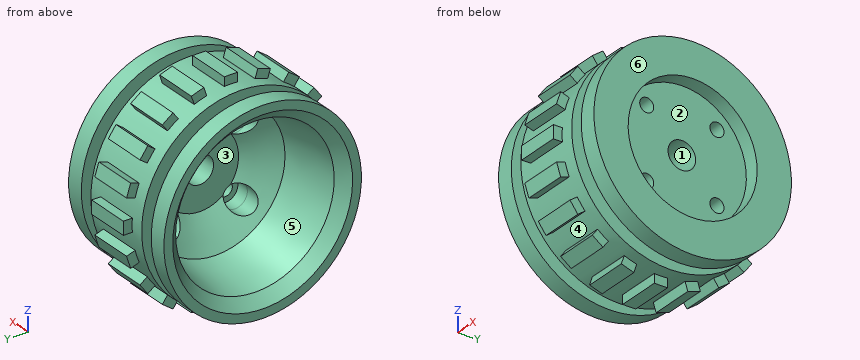
```python
from build123d import *

# Parameters (mm, degrees)
SKETCH_5_R               = 1.6
CUT_EXTRUDE_1_DEPTH      = 42.473606065
SKETCH_6_R               = 2.85
CUT_EXTRUDE_2_DEPTH      = 3
CHAMFER_1_SIZE           = 5
CHAMFER_1_SIZE_2         = 6.164015259
CHAMFER_2_SIZE           = 2
CHAMFER_2_SIZE2          = 2.465606104
SKETCH_8_W               = 3
SKETCH_8_H               = 4
SKETCH_56_W              = 10
SKETCH_56_H              = 3.522984106
EXTRUDE_2_DEPTH          = 1.5
PATTERN_CIRCULAR_2_COUNT = 20


with BuildPart() as part:
    # Эскиз4 → Повернуть1 (revolve)
    with BuildSketch(Plane.XY, mode=Mode.PRIVATE) as revolve_1_sk:
        Polygon((-30, 22.5), (-30, 18.491274218), (-10.2, 15), (-10.2, 3.15), (-3.4, 3.15), (-3.4, 14.7), (0, 14.7), (0, 22.5), align=None)
    revolve(revolve_1_sk.sketch.rotate(Axis((-30, 0, 0), (1, 0, 0)), 90), axis=Axis((-30, 0, 0), (1, 0, 0)))

    # Эскиз5 → Вырез-Вытянуть1 (cut, through all)
    with BuildSketch(Plane(origin=(-3.4, 0, 0), x_dir=(0, 0, -1), z_dir=(1, 0, 0))):
        with Locations((8.000913229, 8.000913229)):
            Circle(SKETCH_5_R)
        with Locations((-8.000913229, 8.000913229)):
            Circle(SKETCH_5_R)
        with Locations((-8.000913229, -8.000913229)):
            Circle(SKETCH_5_R)
        with Locations((8.000913229, -8.000913229)):
            Circle(SKETCH_5_R)
    extrude(amount=-CUT_EXTRUDE_1_DEPTH, mode=Mode.SUBTRACT)

    # Эскиз6 → Вырез-Вытянуть2 (cut)
    with BuildSketch(Plane.ZY.offset(10.2)):
        with Locations((-8.000913229, 8.000913229)):
            Circle(SKETCH_6_R)
        with Locations((8.000913229, 8.000913229)):
            Circle(SKETCH_6_R)
        with Locations((8.000913229, -8.000913229)):
            Circle(SKETCH_6_R)
        with Locations((-8.000913229, -8.000913229)):
            Circle(SKETCH_6_R)
    extrude(amount=-CUT_EXTRUDE_2_DEPTH, mode=Mode.SUBTRACT)

    # Фаска1
    # the kernel refuses this chamfer: 6.164015259, 5 mm, written as the material it adds along each edge
    with BuildSketch(Plane(origin=(-10.2, 0, 0), x_dir=(0, 0, 1), z_dir=(0, 1, 0))) as chamfer_1_piece_1_section:
        Polygon((15 + CHAMFER_1_SIZE * 0.173648177667, -CHAMFER_1_SIZE * 0.984807753012), (15 - CHAMFER_1_SIZE_2, 0), (15, 0), align=None)
    chamfer_1_piece_1 = revolve(axis=Axis((-10.2, 0, 0), (1, 0, 0)), mode=Mode.PRIVATE)
    chamfer_1_piece_1 = chamfer_1_piece_1 - Plane(origin=(-12.574838132, 8.000913229, -8.000913229), x_dir=(0, 0, 1), z_dir=(-1, 0, 0)) * Cylinder(2.85, 64, mode=Mode.PRIVATE)
    chamfer_1_piece_1 = chamfer_1_piece_1 - Plane(origin=(-12.574838132, 8.000913229, 8.000913229), x_dir=(0, 0, 1), z_dir=(-1, 0, 0)) * Cylinder(2.85, 64, mode=Mode.PRIVATE)
    chamfer_1_piece_1 = chamfer_1_piece_1 - Plane(origin=(-12.574838132, -8.000913229, -8.000913229), x_dir=(0, 0, 1), z_dir=(-1, 0, 0)) * Cylinder(2.85, 64, mode=Mode.PRIVATE)
    chamfer_1_piece_1 = chamfer_1_piece_1 - Plane(origin=(-12.574838132, -8.000913229, 8.000913229), x_dir=(0, 0, 1), z_dir=(-1, 0, 0)) * Cylinder(2.85, 64, mode=Mode.PRIVATE)
    add(chamfer_1_piece_1)

    # Фаска2
    chamfer_2_edges = [part.edges().sort_by_distance(p)[0] for p in [
        (-30, 0, -18.491274218),
    ]]
    chamfer_2_side = [part.faces().sort_by_distance(p)[0] for p in [
        (-30, 0, -21.863603897),
    ]]
    chamfer(chamfer_2_edges, length=CHAMFER_2_SIZE, length2=CHAMFER_2_SIZE2, reference=chamfer_2_side[0])

    # Эскиз8 → Вырез-Повернуть1 (revolve, cut)
    with BuildSketch(Plane.XY, mode=Mode.PRIVATE) as cut_revolve_1_sk:
        with Locations((-24.5, 21.5)):
            Rectangle(SKETCH_8_W, SKETCH_8_H)
        with Locations((-5.5, 21.5)):
            Rectangle(SKETCH_8_W, SKETCH_8_H)
    revolve(cut_revolve_1_sk.sketch.rotate(Axis((-30, 0, 0), (1, 0, 0)), 90), axis=Axis((-30, 0, 0), (1, 0, 0)), mode=Mode.SUBTRACT)

    # Эскиз56 → Бобышка-Вытянуть2 (add, symmetric)
    with BuildSketch(Plane.XY):
        with Locations((-15, 22.738507947)):
            Rectangle(SKETCH_56_W, SKETCH_56_H)
    extrude_2 = extrude(amount=EXTRUDE_2_DEPTH, both=True)

    # Круговой массив2: Бобышка-Вытянуть2 ×20 about axis
    pattern_circular_2_axis = Axis((0, 0, 0), (1, 0, 0))
    for i in range(1, PATTERN_CIRCULAR_2_COUNT):
        add(extrude_2.rotate(pattern_circular_2_axis, i * 360 / PATTERN_CIRCULAR_2_COUNT))


solid = part.part
```
For this review, take the finished solid that the model builds, in its own axes (mm). Face numbers are marked on the shaded views. A direction names the side the tool comes from. Round coordinates to 2 decimals unless told otherwise and drop trailing zeros. Write each loop counter-clockwise with the first axis right and the second up, starting at its lowest first coordinate (ties: lowest second). Pieces come first, ordered by that corner, then holes. Notation, with made-up numbers: (73.5, 10.25) -> (82.5, 10.25) arc R23 cw to (82.5, 19.25) -> close; hole circle Ø9 at (79, 10.5). An arc over 180 degrees is marked (long way). One line per question, with ' | ' between items. Start each with the question number.
1) Mouldability with a two-part tool opening along Z and no side actions: class the marked faces 5 and 6 as +Z half, -Z half, draft (parallel to the pull), parting line (faces both ways), or undercut.
2) Add section A-A (x = -6.25). Write out the cut boundary in (y, z).
3) Machinability: for the marked faces 1, 2, 3 and 4, which of the approach directions +Z, -Z, +X, -X, +Y, -Y give a long, thin tool a straight path to every point of the face, cutting with its end or side? Answer none if there is none.
4) For pin 1 Ø10 at (x, z) = (-21, -9) entering from -Y; pin 2 Ø6 at (x, z) = (-18, -16.5) entering from +Y; pin 3 Ø4 at (y, z) = (18.5, -13) entering from -X; pin 4 Ø6 at (y, z) = (6, 2) entering from -X, all flat-tipped, find the tip position at first contact; note any pin that passes through.
5) Wall thickness on line 1 along X through (y, z) = (6, 20); line 2 along Y through (x, z) = (-18.5, -19.5); line 3 along Y through (x, z) = (-7.25, -5.5): over which ranges is each line inside the solid? List them lowest first.
Reported:
1) face 5: undercut | face 6: draft
2) outline: circle Ø39 at (0, 0); hole circle Ø3.2 at (-8, -8); hole circle Ø3.2 at (-8, 8); hole circle Ø6.3 at (0, 0); hole circle Ø3.2 at (8, -8); hole circle Ø3.2 at (8, 8)
3) face 1: +X, -X | face 2: +X | face 3: -X | face 4: none
4) pin 1: stops at y = -23.76 | pin 2: stops at y = 20.48 | pin 3: stops at x = -30 | pin 4: stops at x = -10.54
5) line 1: x = -30 to -26, -23 to -7, -4 to 0 | line 2: y = -14.84 to -12.31, -11.22 to 11.22, 12.31 to 14.84 | line 3: y = -21.82 to -9.37, -6.63 to 6.63, 9.37 to 21.82
